Here's how the part is built. I have some questions about the finished solid (model axes, mm). Face numbers are marked on the shaded views. A direction names the side the tool comes from. Coordinates: 2 decimals unless noted, no trailing zeros. Write each loop counter-clockwise with the first axis right and the second up, starting at its lowest first coordinate (ties: lowest second). Pieces come first, ordered by that corner, then holes. Notation, with made-up numbers: (0.25, 67) -> (13.25, 67) arc R33 ccw to (13.25, 101) -> close; hole circle Ø1 at (20, 14). An arc over 180 degrees is marked (long way). Use a Markdown table: item, result. Add a question column.
Item 1: Imagine slicing it at D-D, the plane y = 14. Write out the boundary of the cut face in (x, z).
Item 2: If I drill on line 1 along Z through (x, y) = (-11.5, 20); line 2 along X through (y, z) = (-1.5, -45); line 3 along X through (y, z) = (4.5, 15), over which ranges is the centre line in solid material (lowest first)? Write a range as from..to.
Item 3: On a 3-axis mill with a long thin cutter (end or side, diameter ignored), from which of +Z, -Z, +X, -X, +Y, -Y can I reach the whole of each face in a straight line? I mean the marked faces 1, 2 and 3. Say none if no direction works.
Item 4: Imagine slicing it at A-A, the plane y = 0. Write out the boundary of the cut face in (x, z).
Item 5: Imagine slicing it at C-C, the plane z = -58. Write out the boundary of the cut face in (x, y), and give its area (3 significant figures).
Item 6: Will these pins go through, and if not, where does the flat tip stop? pin 1 Ø8 at (x, z) = (4.5, -22) entering from +Y; pin 2 Ø6 at (x, y) = (-7.5, 3.5) entering from -Z; pin 3 Ø1.5 at (x, y) = (-8, 23) entering from +Z; pin 4 Ø8 at (x, y) = (20, -9.5) entering from -Z.
```python
from build123d import *

# Parameters (mm, degrees)
F0_R          = 38.1
F1_DEPTH      = 7.62
F3_D          = 12.7
F4_R          = 6.35
F5_DEPTH      = 76.2
F5_DEPTH_BACK = 76.2


with BuildPart() as f1:
    # F0 (on Top) → F1 (new body)
    with BuildSketch(Plane.XY):
        Circle(F0_R)
    extrude(amount=F1_DEPTH)

    # F3 (through all)
    with Locations(Plane(origin=(0, 0, 0), x_dir=(1, 0, 0), z_dir=(0, 0, -1))):
        with Locations((0, 0)):
            Hole(F3_D / 2)

    # F4 (on Top) → F5 (join, two sides)
    with BuildSketch(Plane.XY) as f5_sk:
        Circle(F4_R)
    extrude(amount=F5_DEPTH)
    extrude(f5_sk.sketch, amount=-F5_DEPTH_BACK)


solid = f1.part
```
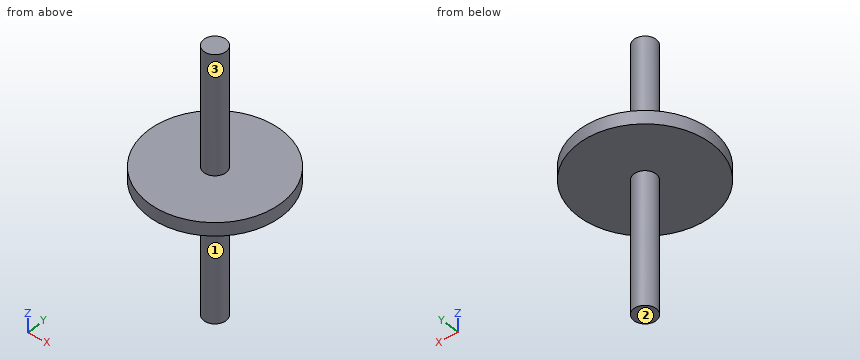
Ans:
| question | item | result |
|---|---|---|
| 1 | outline | (-35.43, 0) -> (35.43, 0) -> (35.43, 7.62) -> (-35.43, 7.62) -> close |
| 2 | line 1 | z = 0..7.62 |
| 2 | line 2 | x = -6.17..6.17 |
| 2 | line 3 | x = -4.48..4.48 |
| 3 | face 1 | -Z |
| 3 | face 2 | -Z, +X, -X, +Y, -Y |
| 3 | face 3 | +Z |
| 4 | outline | (-38.1, 0) -> (-6.35, 0) -> (-6.35, -76.2) -> (6.35, -76.2) -> (6.35, 0) -> (38.1, 0) -> (38.1, 7.62) -> (6.35, 7.62) -> (6.35, 76.2) -> (-6.35, 76.2) -> (-6.35, 7.62) -> (-38.1, 7.62) -> close |
| 5 | outline | circle Ø12.7 at (0, 0) |
| 5 | area | 127 mm^2 |
| 6 | pin 1 | stops at y = 6.33 |
| 6 | pin 2 | stops at z = -76.2 |
| 6 | pin 3 | stops at z = 7.62 |
| 6 | pin 4 | stops at z = 0 |
